```python
from build123d import *

# Parameters (mm, degrees)
SKETCH1_W               = 154
SKETCH1_H               = 86
BOSS_EXTRUDE1_DEPTH     = 0.635
SKETCH2_R               = 2.248
CUT_EXTRUDE3_DEPTH      = 342.301440511
LPATTERN1_COUNT         = 5
LPATTERN1_PITCH         = 88.5
SKETCH3_R               = 2.248
CUT_EXTRUDE5_DEPTH      = 342.301440511
LPATTERN2_COUNT         = 6
LPATTERN2_PITCH         = 60
MIRROR1_COPY_1_SKETCH_R = 2.248
MIRROR1_COPY_1_DEPTH    = 342.301440511
MIRROR1_COPY_2_SKETCH_R = 2.248
MIRROR1_COPY_2_DEPTH    = 342.301440511
MIRROR1_COPY_3_SKETCH_R = 2.248
MIRROR1_COPY_3_DEPTH    = 342.301440511
MIRROR1_COPY_4_SKETCH_R = 2.248
MIRROR1_COPY_4_DEPTH    = 342.301440511
MIRROR1_COPY_5_SKETCH_R = 2.248
MIRROR1_COPY_5_DEPTH    = 342.301440511


with BuildPart() as part:
    # Sketch1 → Boss-Extrude1 (new body)
    with BuildSketch(Plane.XY):
        Polygon((-283.600620106, 189.886698706), (-283.600620106, 74.886698706), (-13.600620106, 74.886698706), (-13.600620106, -90.113301294), (-283.600620106, -90.113301294), (-283.600620106, -110.113301294), (170.399379894, -110.113301294), (170.399379894, 189.886698706), align=None)
        with Locations((78.399379894, 31.886698706)):
            Rectangle(SKETCH1_W, SKETCH1_H, mode=Mode.SUBTRACT)
    extrude(amount=BOSS_EXTRUDE1_DEPTH)

    # Sketch2 → Cut-Extrude3 (cut, through all)
    with BuildSketch(Plane.XY):
        with Locations((-233.600620106, 181.911698706)):
            Circle(SKETCH2_R)
    cut_extrude3 = extrude(amount=CUT_EXTRUDE3_DEPTH, mode=Mode.SUBTRACT)

    # LPattern1: Cut-Extrude3 ×5
    with Locations(*[(i * LPATTERN1_PITCH, 0, 0) for i in range(1, LPATTERN1_COUNT)]):
        add(cut_extrude3, mode=Mode.SUBTRACT)

    # Sketch3 → Cut-Extrude5 (cut, through all)
    with BuildSketch(Plane.XY):
        with Locations((-275.625620106, 159.886698706)):
            Circle(SKETCH3_R)
    cut_extrude5 = extrude(amount=CUT_EXTRUDE5_DEPTH, mode=Mode.SUBTRACT)

    # LPattern2: Cut-Extrude5 ×6
    with Locations(*[(0, -i * LPATTERN2_PITCH, 0) for i in range(1, LPATTERN2_COUNT)]):
        add(cut_extrude5, mode=Mode.SUBTRACT)

    # Mirror1: Cut-Extrude5 across plane
    add(cut_extrude5.mirror(Plane.ZY.offset(56.600620106)), mode=Mode.SUBTRACT)

    # Mirror1 copy 1 sketch → Mirror1 copy 1 (cut, through all)
    with BuildSketch(Plane(origin=(-113.201240213, -60, 0), x_dir=(-1, 0, 0), z_dir=(0, 0, 1))):
        with Locations((-275.625620106, -159.886698706)):
            Circle(MIRROR1_COPY_1_SKETCH_R)
    extrude(amount=MIRROR1_COPY_1_DEPTH, mode=Mode.SUBTRACT)

    # Mirror1 copy 2 sketch → Mirror1 copy 2 (cut, through all)
    with BuildSketch(Plane(origin=(-113.201240213, -120, 0), x_dir=(-1, 0, 0), z_dir=(0, 0, 1))):
        with Locations((-275.625620106, -159.886698706)):
            Circle(MIRROR1_COPY_2_SKETCH_R)
    extrude(amount=MIRROR1_COPY_2_DEPTH, mode=Mode.SUBTRACT)

    # Mirror1 copy 3 sketch → Mirror1 copy 3 (cut, through all)
    with BuildSketch(Plane(origin=(-113.201240213, -180, 0), x_dir=(-1, 0, 0), z_dir=(0, 0, 1))):
        with Locations((-275.625620106, -159.886698706)):
            Circle(MIRROR1_COPY_3_SKETCH_R)
    extrude(amount=MIRROR1_COPY_3_DEPTH, mode=Mode.SUBTRACT)

    # Mirror1 copy 4 sketch → Mirror1 copy 4 (cut, through all)
    with BuildSketch(Plane(origin=(-113.201240213, -240, 0), x_dir=(-1, 0, 0), z_dir=(0, 0, 1))):
        with Locations((-275.625620106, -159.886698706)):
            Circle(MIRROR1_COPY_4_SKETCH_R)
    extrude(amount=MIRROR1_COPY_4_DEPTH, mode=Mode.SUBTRACT)

    # Mirror1 copy 5 sketch → Mirror1 copy 5 (cut, through all)
    with BuildSketch(Plane(origin=(-113.201240213, -300, 0), x_dir=(-1, 0, 0), z_dir=(0, 0, 1))):
        with Locations((-275.625620106, -159.886698706)):
            Circle(MIRROR1_COPY_5_SKETCH_R)
    extrude(amount=MIRROR1_COPY_5_DEPTH, mode=Mode.SUBTRACT)


solid = part.part
```
Work out the finished part from the listing and answer in its coordinate system (mm). Coordinates: 2 decimals unless noted, no trailing zeros. Write each loop counter-clockwise with the first axis right and the second up, starting at its lowest first coordinate (ties: lowest second). Pieces come first, ordered by that corner, then holes.
Q1. A cutting plane is placed at B-B, the plane x = -19. Give the vertices of the cut face in (y, z) (3 decimals).
Q2. A cutting plane is placed at C-C, the plane z = 0.15. State how many separate pieces and enclosed holes the cut face has, then the cut area to 3 significant figures.
Q3. A cutting plane is placed at A-A, the plane y = -2.5. Give the vertices of the cut face in (x, z) (3 decimals).
Q4. Find the intervals of material crossed by line 1 (Y direction, x = -22, z = 0.5); line 2 (Y direction, x = 145, z = 0.5); line 3 (X direction, y = 17.5, z = 0.3), in increasing order.
Findings below:
1. outline: (-110.113, 0) - (-90.113, 0) - (-90.113, 0.635) - (-110.113, 0.635) - close; (74.887, 0) - (189.887, 0) - (189.887, 0.635) - (74.887, 0.635) - close
2. separate pieces: 1
2. enclosed holes: 13
2. area: 78,200 mm2
3. outline: (-13.601, 0) - (1.399, 0) - (1.399, 0.635) - (-13.601, 0.635) - close; (155.399, 0) - (170.399, 0) - (170.399, 0.635) - (155.399, 0.635) - close
4. line 1: y = -110.11 to -90.11, 74.89 to 189.89
4. line 2: y = -110.11 to -11.11, 74.89 to 189.89
4. line 3: x = -13.6 to 1.4, 155.4 to 170.4
